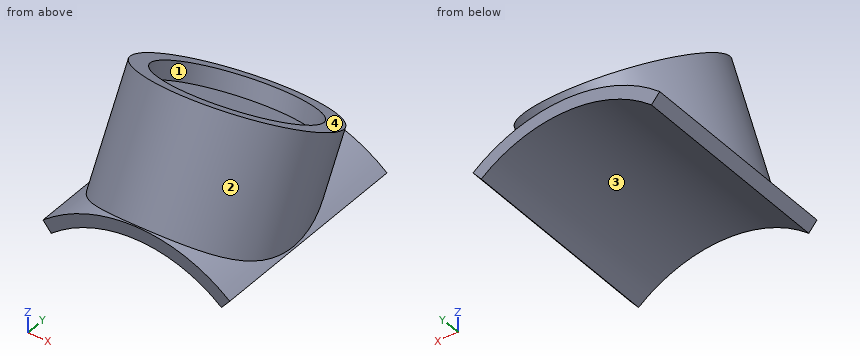
Autodesk Inventor part; units mm, degrees
ref_plane "Work Plane1" through (0, -10.7781, 26.0195) normal (0, -0.5, -0.866) x (1, 0, 0)
ref_plane "YZ Plane" through (0, 0, 0) normal (1, 0, 0) x (0, 1, 0)
ref_plane "XZ Plane" through (0, 0, 0) normal (0, 1, 0) x (-1, 0, 0)
sketch "Sketch1" plane through (0, 0, 0) normal (1, 0, 0) x (0, 1, 0)
  line L0 (22.9037, 13.0375) -> (-26.2512, 13.0375)
  line L1 (-26.2512, 13.0375) -> (-26.2512, -17.8825)
  line L2 (-26.2512, -17.8825) -> (22.9037, -17.8825)
  line L3 (22.9037, -17.8825) -> (22.9037, 13.0375)
  line L4 (-27.7512, 14.5375) -> (24.4037, 14.5375)
  line L5 (24.4037, 14.5375) -> (24.4037, -19.3825)
  line L6 (24.4037, -19.3825) -> (-27.7512, -19.3825)
  line L7 (-27.7512, -19.3825) -> (-27.7512, 14.5375)
  line L8 (14.8755, 31.453) -> (106.1225, 31.453) construction
  line L9 (5.1094, 14.5375) -> (-10.0461, 23.2875)
  line L10 (-10.0461, 23.2875) -> (-9.0461, 25.0195)
  line L11 (-9.0461, 25.0195) -> (-10.7781, 26.0195)
  line L12 (-10.7781, 26.0195) -> (-17.4073, 14.5375)
  line L13 (24.4037, -2.4225) -> (-27.7512, -2.4225)
  point P0 (0, 0)
  point P1 (22.9037, -2.4225)
  point P2 (-26.2512, -2.4225)
  dimension "d0" = 30.92
  dimension "d1" = 1.5
  dimension "d3" = 17.5
  dimension "d4" = 2
  dimension "d5" = 2
ref_plane "Work Plane1" through (0, -10.7781, 26.0195) normal (0, -0.5, -0.866) x (1, 0, 0)
sketch "Sketch2" plane through (0, -10.7781, 26.0195) normal (0, -0.5, -0.866) x (1, 0, 0)
  line L0 (0, -19.5) -> (0, -2)
  circle A0 centre (0, -10.75) radius 8.75
  circle A1 centre (0, -10.75) radius 10.75
  point P0 (0, -22.3439)
  point P1 (0, 0)
extrude "Extrusion1" add sketch "Sketch2" along normal blind 19 contours A0 L0 | L0 A0 | A1
extrude "Extrusion2" cut sketch "Sketch2" along normal blind 2 contours A0 L0 | L0 A0
revolve "Revolution1" add sketch "Sketch1" angle 360 about axis through (0, 24.4037, -2.4225) along (0, -1, 0) contours L0 L1 L13 L7 L4 L5 L3
sketch "Sketch3" plane through (0, 24.4037, -2.4225) normal (0, 1, 0) x (1, 0, 0)
  circle A0 centre (0, 0) radius 15.46
  circle A1 centre (0, 0) radius 16.96
  point P0 (0, -2.4225)
extrude "Extrusion3" cut sketch "Sketch3" against normal blind 127.25 contours A0
sketch "Sketch4" plane through (0, 0, 0) normal (1, 0, 0) x (0, 1, 0)
  line L0 (24.4037, 14.5375) -> (-27.7512, 14.5375)
  line L1 (7.5764, 14.5375) -> (27.5764, 14.5375)
  line L2 (27.5764, 14.5375) -> (27.5764, -29.1021)
  line L3 (27.5764, -29.1021) -> (7.5764, -29.1021)
  line L4 (7.5764, -29.1021) -> (7.5764, 14.5375)
  line L5 (-17.5694, 14.5375) -> (-31.1808, 14.5375)
  line L6 (-31.1808, 14.5375) -> (-31.1808, -26.5715)
  line L7 (-31.1808, -26.5715) -> (-17.5694, -26.5715)
  line L8 (-17.5694, -26.5715) -> (-17.5694, 14.5375)
  point P0 (0, 0)
  dimension "d21" = 20
extrude "Extrusion4" cut sketch "Sketch4" along normal mid plane 127.25
sketch "Sketch5" plane through (0, 7.5764, -2.4225) normal (0, 1, 0) x (1, 0, 0)
  circle A0 centre (0, 0) radius 16.96
  line L0 (0, 0) -> (-17.0449, -20.3133)
  line L1 (0, 0) -> (26.5172, 0) construction
  line L2 (0, 0) -> (19.6818, -23.4558)
  line L3 (0, 0) -> (30.6194, 0) construction
  arc A1 (19.6818, -23.4558) -> (-16.96, -20.2121) centre (3.3753, 0.9216) ccw
  dimension "d17" = 130
  dimension "d18" = 50
extrude "Extrusion6" cut sketch "Sketch5" against normal blind 127.25 contours A0 L2 L0 | A0 L0 A1 L2 picked at (-8.1801, -7.6911)
properties part number "1'' copper pipe 60 deg mount"
Design review of the part built by this model. Coordinates are the model's own, in mm. Face numbers are marked on the shaded views. Give positions to 0.01 mm unless a question says otherwise; leave off trailing zeros. Loops run counter-clockwise (first coordinate to the right, second up) from the corner with the lowest first, then second, coordinate; pieces in that order, holes last. Notation, with made-up numbers: (-7, 67.25) - (44, 67.25) arc R12 ccw to (44, 80.25) - close; hole circle Ø9 at (56.25, 68). An arc over 180 degrees is marked (long way). Use CSV: the item, a comma, the result in double quotes. Start each with the question number.
1. Insertion check: P1, Ø1.5, axis at y = -6, z = 22, coming from the +X side; P2, Ø8, axis at y = -5.5, z = 19, coming from the +X side; P3, Ø6, axis at x = 4.5, y = -12.5, coming from the -Z side; P4, Ø2.5, axis at x = 2.5, z = 11.5, coming from the +Y side. Each pin has a flat end and moves straight along its axis. Give the tip position at first contact, or say it passes through.
2. Add section A-A (x = -0.5). State the section outline as (y, z) points.
3. Add section B-B (x = -4.5). State the section outline as (y, z) points.
4. Wall thickness on L1, parallel to Y at x = -4, z = 14; L2, parallel to X at y = 4.5, z = 15.75; L3, parallel to Z at x = 2.25, y = -1: over which ranges is each line inside the solid? List them lowest first.
5. Draft analysis for pull direction Y (two halves, no side actions). For the marked faces 1, 2, 3 and 4, state which applies: released by +Y, released by -Y, zero draft, split by the parting line, or undercut.
Results found:
1,P1,"stops at x = 10.04"
1,P2,"stops at x = 10.75"
1,P3,"stops at z = 11.1"
1,P4,"passes through"
2,outline,"(-17.57, 13.03) - (7.58, 13.03) - (7.58, 14.53) - (7.4, 14.53) - (7.83, 15.28) - (6.1, 16.28) - (5.1, 14.54) - (-10.03, 23.28) - (-9.03, 25.01) - (-10.77, 26.01) - (-17.4, 14.53) - (-17.57, 14.53) - close"
3,outline,"(-17.57, 12.37) - (7.58, 12.37) - (7.58, 13.93) - (5.93, 13.93) - (6.99, 15.76) - (5.03, 16.89) - (4.03, 15.16) - (-8.97, 22.66) - (-7.97, 24.4) - (-9.92, 25.53) - (-16.62, 13.93) - (-17.57, 13.93) - close"
4,L1,"y = -17.57 to 7.58"
4,L2,"x = -7.59 to -4.31, 4.31 to 7.59"
4,L3,"z = 12.87 to 18.06"
5,face 1,"undercut"
5,face 2,"split by the parting line"
5,face 3,"zero draft"
5,face 4,"released by +Y"
